Design review of the part built by this model. Coordinates are the model's own, in mm. A direction names the side the tool comes from. Coordinates: 2 decimals unless noted, no trailing zeros. Order: outer loops, then holes, each group sorted by start corner. A loop starts at its lowest first (then second) coordinate and runs counter-clockwise, first axis right, second up. Notation, with made-up numbers: (38, 78.25) -> (56, 78.25) arc R28 ccw to (56, 107.25) -> close; hole circle Ø7 at (49.25, -26.5). An arc over 180 degrees is marked (long way). Use a Markdown table: item, result. Add a question column.
Q1. The part is to be moulded in two halves that separate along X. For faces 1 (the face through (-63.497, -0.056, 0.279)), 2 (the face through (-30.51, -0.056, -17.434)), 3 (the face through (-17.434, -0.056, 30.51)), 4 (the face through (-0.279, -0.056, -63.497)), say which applies: pulls with the +X half, pulls with the -X half, needs draft (parallel to the pull), parting line crosses it, or undercut.
Q2. Insertion check: pin 1 (1 mm diameter, centred on x = 22.5, y = -1, fed in from +Z); pin 2 (2 mm diameter, centred on x = -24.5, y = 2.5, fed in from +Z); pin 3 (2 mm diameter, centred on y = 2.5, z = -18, fed in from +X). Each pin has a flat end and moves straight along its axis. Give the tip position at first contact, or say it passes through.
Q3. Add section C-C (z = 3.5). State the section outline as (x, y) points, then the cut area to 3 significant figures.
Q4. Machinability: for faces 5 (the face through (0.279, -0.056, 63.497)), 6 (the face through (-9.246, -0.056, -33.901)), which of the approach directions +Z, -Z, +X, -X, +Y, -Y give a long, thin tool a straight path to every point of the face, cutting with its end or side? Answer none if there is none.
Q5. Add section D-D (x = 2). State the section outline as (y, z) points.
Q6. Add section A-A (x = 33.5). State the section outline as (y, z) points.
Q7. Wall thickness on probe 1 along Z at (x, y) = (-26.5, 0.75); probe 2 along Z at (x, y) = (-31, -3); probe 3 along X at (y, z) = (-2.5, 51.5): over which ranges is each line inside the solid? List them lowest first.
Q8. Add section B-B (z = -32). State the section outline as (x, y) points, then the cut area to 3 significant figures.
from build123d import *

# Parameters (mm, degrees)
F0_R     = 10.6172
F1_DEPTH = 3.9751
F2_R     = 1.27


with BuildPart() as f1:
    # F0 (on Front) → F1 (new body, symmetric)
    with BuildSketch(Plane.XZ):
        with BuildLine():
            Line((11.0363, -4.5713851384), (11.0363, 0))
            ThreePointArc((11.0363, 0), (10.1962116818, -4.2234091715), (7.8038425587, -7.8038425798))
            Line((7.8038425587, -7.8038425798), (11.0363, -4.5713851384))
        make_face()
        with BuildLine():
            ThreePointArc((7.8038425896, 7.8038425488), (10.1962116902, 4.2234091513), (11.0363, 0))
            Line((11.0363, 0), (11.0363, 4.5713851384))
            Line((11.0363, 4.5713851384), (7.8038425896, 7.8038425488))
        make_face()
        with BuildLine():
            Line((11.0363, 4.5713851384), (11.0363, 0))
            Line((11.0363, 0), (11.0363, -4.5713851384))
            Line((11.0363, -4.5713851384), (50.8, -12.7))
            ThreePointArc((50.8, -12.7), (63.5, 0), (50.8, 12.7))
            Line((50.8, 12.7), (11.0363, 4.5713851384))
        make_face()
        with Locations((50.8, 0)):
            Circle(F0_R, mode=Mode.SUBTRACT)
        with BuildLine():
            ThreePointArc((0, 11.0363), (4.2234091779, 10.1962116791), (7.8038425896, 7.8038425488))
            Line((7.8038425896, 7.8038425488), (4.5713851384, 11.0363))
            Line((4.5713851384, 11.0363), (0, 11.0363))
        make_face()
        with BuildLine():
            Line((4.5713851384, 11.0363), (7.8038425896, 7.8038425488))
            Line((7.8038425896, 7.8038425488), (11.0363, 4.5713851384))
            Line((11.0363, 4.5713851384), (44.9012806053, 26.9407683632))
            ThreePointArc((44.9012806053, 26.9407683632), (44.9012806053, 44.9012806053), (26.9407683632, 44.9012806053))
            Line((26.9407683632, 44.9012806053), (4.5713851384, 11.0363))
        make_face()
        with Locations((35.9210244843, 35.9210244843)):
            Circle(F0_R, mode=Mode.SUBTRACT)
        with BuildLine():
            Line((4.5713851384, -11.0363), (7.8038425587, -7.8038425798))
            ThreePointArc((7.8038425587, -7.8038425798), (4.2234091577, -10.1962116875), (0, -11.0363))
            Line((0, -11.0363), (4.5713851384, -11.0363))
        make_face()
        with BuildLine():
            Line((11.0363, -4.5713851384), (7.8038425587, -7.8038425798))
            Line((7.8038425587, -7.8038425798), (4.5713851384, -11.0363))
            Line((4.5713851384, -11.0363), (26.9407683632, -44.9012806053))
            ThreePointArc((26.9407683632, -44.9012806053), (44.9012806053, -44.9012806053), (44.9012806053, -26.9407683632))
            Line((44.9012806053, -26.9407683632), (11.0363, -4.5713851384))
        make_face()
        with Locations((35.9210244843, -35.9210244843)):
            Circle(F0_R, mode=Mode.SUBTRACT)
        with BuildLine():
            ThreePointArc((-7.8038425634, 7.803842575), (-4.2234091608, 10.1962116862), (0, 11.0363))
            Line((0, 11.0363), (-4.5713851384, 11.0363))
            Line((-4.5713851384, 11.0363), (-7.8038425634, 7.803842575))
        make_face()
        with BuildLine():
            Line((-4.5713851384, 11.0363), (0, 11.0363))
            Line((0, 11.0363), (4.5713851384, 11.0363))
            Line((4.5713851384, 11.0363), (12.7, 50.8))
            ThreePointArc((12.7, 50.8), (0, 63.5), (-12.7, 50.8))
            Line((-12.7, 50.8), (-4.5713851384, 11.0363))
        make_face()
        with Locations((0, 50.8)):
            Circle(F0_R, mode=Mode.SUBTRACT)
        with BuildLine():
            Line((-4.5713851384, -11.0363), (0, -11.0363))
            ThreePointArc((0, -11.0363), (-4.2234091646, -10.1962116847), (-7.8038425692, -7.8038425692))
            Line((-7.8038425692, -7.8038425692), (-4.5713851384, -11.0363))
        make_face()
        with BuildLine():
            Line((4.5713851384, -11.0363), (0, -11.0363))
            Line((0, -11.0363), (-4.5713851384, -11.0363))
            Line((-4.5713851384, -11.0363), (-12.7, -50.8))
            ThreePointArc((-12.7, -50.8), (0, -63.5), (12.7, -50.8))
            Line((12.7, -50.8), (4.5713851384, -11.0363))
        make_face()
        with Locations((0, -50.8)):
            Circle(F0_R, mode=Mode.SUBTRACT)
        with BuildLine():
            ThreePointArc((-11.0363, 0), (-10.1962116831, 4.2234091684), (-7.8038425634, 7.803842575))
            Line((-7.8038425634, 7.803842575), (-11.0363, 4.5713851384))
            Line((-11.0363, 4.5713851384), (-11.0363, 0))
        make_face()
        with BuildLine():
            Line((-11.0363, 4.5713851384), (-7.8038425634, 7.803842575))
            Line((-7.8038425634, 7.803842575), (-4.5713851384, 11.0363))
            Line((-4.5713851384, 11.0363), (-26.9407683632, 44.9012806053))
            ThreePointArc((-26.9407683632, 44.9012806053), (-44.9012806053, 44.9012806053), (-44.9012806053, 26.9407683632))
            Line((-44.9012806053, 26.9407683632), (-11.0363, 4.5713851384))
        make_face()
        with Locations((-35.9210244843, 35.9210244843)):
            Circle(F0_R, mode=Mode.SUBTRACT)
        with BuildLine():
            Line((-11.0363, -4.5713851384), (-7.8038425692, -7.8038425692))
            ThreePointArc((-7.8038425692, -7.8038425692), (-10.1962116847, -4.2234091646), (-11.0363, 0))
            Line((-11.0363, 0), (-11.0363, -4.5713851384))
        make_face()
        with BuildLine():
            Line((-4.5713851384, -11.0363), (-7.8038425692, -7.8038425692))
            Line((-7.8038425692, -7.8038425692), (-11.0363, -4.5713851384))
            Line((-11.0363, -4.5713851384), (-44.9012806053, -26.9407683632))
            ThreePointArc((-44.9012806053, -26.9407683632), (-44.9012806053, -44.9012806053), (-26.9407683632, -44.9012806053))
            Line((-26.9407683632, -44.9012806053), (-4.5713851384, -11.0363))
        make_face()
        with Locations((-35.9210244843, -35.9210244843)):
            Circle(F0_R, mode=Mode.SUBTRACT)
        with BuildLine():
            Line((-11.0363, -4.5713851384), (-11.0363, 0))
            Line((-11.0363, 0), (-11.0363, 4.5713851384))
            Line((-11.0363, 4.5713851384), (-50.8, 12.7))
            ThreePointArc((-50.8, 12.7), (-63.5, 0), (-50.8, -12.7))
            Line((-50.8, -12.7), (-11.0363, -4.5713851384))
        make_face()
        with Locations((-50.8, 0)):
            Circle(F0_R, mode=Mode.SUBTRACT)
    extrude(amount=F1_DEPTH, both=True)

    # F2
    f2_edges = [f1.edges().sort_by_distance(p)[0] for p in [
        (4.571385, 0, 11.0363),
        (-4.571385, 0, 11.0363),
        (-11.0363, 0, 4.571385),
        (-11.0363, 0, -4.571385),
        (-4.571385, 0, -11.0363),
        (4.571385, 0, -11.0363),
        (11.0363, 0, -4.571385),
        (11.0363, 0, 4.571385),
    ]]
    fillet(f2_edges, radius=F2_R)


solid = f1.part
Established:
| question | item | result |
|---|---|---|
| 1 | face 1 | pulls with the -X half |
| 1 | face 2 | undercut |
| 1 | face 3 | undercut |
| 1 | face 4 | parting line crosses it |
| 2 | pin 1 | z = 38.94 |
| 2 | pin 2 | z = 42.72 |
| 2 | pin 3 | x = 32.88 |
| 3 | outline | (-63.01, -3.98) -> (-60.82, -3.98) -> (-60.82, 3.98) -> (-63.01, 3.98) -> close; (-40.78, -3.98) -> (-10.47, -3.98) -> (-10.47, 3.98) -> (-40.78, 3.98) -> close; (10.47, -3.98) -> (40.78, -3.98) -> (40.78, 3.98) -> (10.47, 3.98) -> close; (60.82, -3.98) -> (63.01, -3.98) -> (63.01, 3.98) -> (60.82, 3.98) -> close |
| 3 | area | 517 mm^2 |
| 4 | face 5 | +Z, +Y, -Y |
| 4 | face 6 | +Y, -Y |
| 5 | outline | (-3.98, -63.34) -> (3.98, -63.34) -> (3.98, -61.23) -> (-3.98, -61.23) -> close; (-3.98, -40.37) -> (3.98, -40.37) -> (3.98, -10.85) -> (-3.98, -10.85) -> close; (-3.98, 10.85) -> (3.98, 10.85) -> (3.98, 40.37) -> (-3.98, 40.37) -> close; (-3.98, 61.23) -> (3.98, 61.23) -> (3.98, 63.34) -> (-3.98, 63.34) -> close |
| 6 | outline | (-3.98, -48.39) -> (3.98, -48.39) -> (3.98, -46.26) -> (-3.98, -46.26) -> close; (-3.98, -25.58) -> (3.98, -25.58) -> (3.98, -19.41) -> (-3.98, -19.41) -> close; (-3.98, -9.16) -> (3.98, -9.16) -> (3.98, 9.16) -> (-3.98, 9.16) -> close; (-3.98, 19.41) -> (3.98, 19.41) -> (3.98, 25.58) -> (-3.98, 25.58) -> close; (-3.98, 46.26) -> (3.98, 46.26) -> (3.98, 48.39) -> (-3.98, 48.39) -> close |
| 7 | probe 1 | -44.23 to -40.82, -31.03 to -14.79, -7.73 to 7.73, 14.79 to 31.03, 40.82 to 44.23 |
| 7 | probe 2 | -47.63 to -45.33, -26.51 to -17.76, -8.65 to 8.65, 17.76 to 26.51, 45.33 to 47.63 |
| 7 | probe 3 | -12.68 to -10.59, 10.59 to 12.68 |
| 8 | outline | (-48, -3.98) -> (-45.79, -3.98) -> (-45.79, 3.98) -> (-48, 3.98) -> close; (-26.05, -3.98) -> (-18.42, -3.98) -> (-18.42, 3.98) -> (-26.05, 3.98) -> close; (-8.86, -3.98) -> (8.86, -3.98) -> (8.86, 3.98) -> (-8.86, 3.98) -> close; (18.42, -3.98) -> (26.05, -3.98) -> (26.05, 3.98) -> (18.42, 3.98) -> close; (45.79, -3.98) -> (48, -3.98) -> (48, 3.98) -> (45.79, 3.98) -> close |
| 8 | area | 297 mm^2 |
